Read the model definition and answer for the solid it produces. Units are mm, in the model's axes. A direction names the side the tool comes from. Give positions to 0.01 mm unless a question says otherwise; leave off trailing zeros. Write each loop counter-clockwise with the first axis right and the second up, starting at its lowest first coordinate (ties: lowest second). Pieces come first, ordered by that corner, then holes. Notation, with made-up numbers: M 51.25,-12 L 62.25,-12 A24 cw 62.25,26 Z; hole C 20.25,2 d3. An arc over 180 degrees is marked long. Use a Markdown table: item, result. Add a question column.
Item 1: Consider probe 1 along X at (y, z) = (-6.5, -1.25); probe 2 along X at (y, z) = (-8.5, 7); probe 3 along Y at (x, z) = (-1.5, 10.75) (3 decimals). Determine where each line is inside the solid, lowest interval first. Write a range as [from, to].
Item 2: A cutting plane is placed at B-B on y = 0. Determine the outline of the cut face in (x, z) (3 decimals).
Item 3: A cutting plane is placed at D-D on x = 9. Determine the outline of the cut face in (y, z).
Item 4: For faces 1 (the flat face through (0, -5, 0)), 2 (the flat face through (56.134, 9, -6)), 3 (the flat face through (66.294, 0, 0)), determine the directions among +Z, -Z, +X, -X, +Y, -Y from which every point of the face is accessible in a straight line to the end or side of a thin tool.
Item 5: A cutting plane is placed at C-C on x = -6.5. Determine the outline of the cut face in (y, z) (3 decimals).
Item 6: A cutting plane is placed at A-A on z = 0. Determine the outline of the cut face in (x, y) (3 decimals).
Item 7: Given P1, Ø6, axis at x = 8, z = 1.5, coming from the -Y side; P2, Ø5, axis at x = 40, y = -9, coming from the -Z side; P3, Ø12, axis at x = 10.5, y = 9.5, coming from the -Z side; P4, Ø3, axis at y = -7, z = 11.5, coming from the -X side, each flat-ended and moving along its own axis, determine where each tip first touches the part or whether it passes through.
Item 8: The mould has two halves that part along X. Classify faces 4 (the flat face through (-4.149, -0.044, -6.626)), 5 (the cylindrical face through (60.52, -12.4, -2.75)), 6 (the cylindrical face through (-3.626, 0.044, 0.954)): pulls with the +X half, pulls with the -X half, needs draft (parallel to the pull), parting line crosses it, or undercut.
from build123d import *

# Parameters (mm, degrees)
F0_W     = 5.842
F0_H     = 12.7
F0_R     = 3.175
F2_DEPTH = 3.175
F3_R     = 1.27


with BuildPart() as f1:
    # F0 (on Front) → F1 (revolve)
    with BuildSketch(Plane.XZ):
        with Locations((2.921, 6.35)):
            Rectangle(F0_W, F0_H)
        Polygon((5.842, 12.7), (5.842, 0), (66.294, 0), (66.294, 12.7), (56.134, 12.7), (56.134, 10.16), (10.16, 10.16), (10.16, 12.7), align=None)
    revolve(axis=Axis((33.147, 0, 0), (-1, 0, 0)))

    # F0 (on Front) → F2 (join, symmetric)
    with BuildSketch(Plane.XZ):
        with BuildLine():
            Line((-0.9398, 0), (0, 0))
            Line((0, 0), (0, 12.7))
            Line((0, 12.7), (5.842, 12.7))
            Line((5.842, 12.7), (5.842, 15.24))
            Line((5.842, 15.24), (-0.508, 15.24))
            Line((-0.508, 15.24), (-10.88063, 3.847543))
            ThreePointArc((-10.88063, 3.847543), (-4.591961, 5.329721), (-0.9398, 0))
        make_face()
        with BuildLine():
            ThreePointArc((-8.182663, -5.506983), (-3.195791, -4.549339), (-0.9398, 0))
            ThreePointArc((-0.9398, 0), (-4.591961, 5.329721), (-10.88063, 3.847543))
            ThreePointArc((-10.88063, 3.847543), (-12.145978, -1.583727), (-8.182663, -5.506983))
        make_face()
        with Locations((-6.6548, 0)):
            Circle(F0_R, mode=Mode.SUBTRACT)
        with BuildLine():
            Line((5.842, 0), (0, 0))
            Line((0, 0), (-0.9398, 0))
            ThreePointArc((-0.9398, 0), (-3.195791, -4.549339), (-8.182663, -5.506983))
            Line((-8.182663, -5.506983), (5.842, -9.398))
            Line((5.842, -9.398), (5.842, 0))
        make_face()
        with Locations((2.921, 6.35)):
            Rectangle(F0_W, F0_H)
    extrude(amount=F2_DEPTH, both=True)

    # F3
    f3_edges = [f1.edges().sort_by_distance(p)[0] for p in [
        (66.294, 0, -12.7),
    ]]
    fillet(f3_edges, radius=F3_R)


solid = f1.part
Filled in:
| question | item | result |
|---|---|---|
| 1 | probe 1 | [0, 66.29] |
| 1 | probe 2 | [0, 10.16], [56.13, 66.29] |
| 1 | probe 3 | [-3.175, 3.175] |
| 2 | outline | M -10.881,3.848 A5.715 ccw -8.183,-5.507 L 0,-7.777 L 0,-12.7 L 10.16,-12.7 L 10.16,-10.16 L 56.134,-10.16 L 56.134,-12.7 L 65.024,-12.7 A1.27 ccw 66.294,-11.43 L 66.294,11.43 A1.27 ccw 65.024,12.7 L 56.134,12.7 L 56.134,10.16 L 10.16,10.16 L 10.16,12.7 L 5.842,12.7 L 5.842,15.24 L -0.508,15.24 Z; hole C -6.655,0 d6.35 |
| 3 | outline | C 0,0 d25.4 |
| 4 | face 1 | -Z, -X |
| 4 | face 2 | none |
| 4 | face 3 | +Z, -Z, +X, +Y, -Y |
| 5 | outline | M -3.175,-5.974 L 3.175,-5.974 L 3.175,-3.171 L -3.175,-3.171 Z; M -3.175,3.171 L 3.175,3.171 L 3.175,8.659 L -3.175,8.659 Z |
| 6 | outline | M -12.37,-3.175 L -9.83,-3.175 L -9.83,3.175 L -12.37,3.175 Z; M -3.48,-3.175 L 0,-3.175 L 0,-12.7 L 10.16,-12.7 L 10.16,-10.16 L 56.134,-10.16 L 56.134,-12.7 L 65.024,-12.7 A1.27 ccw 66.294,-11.43 L 66.294,11.43 A1.27 ccw 65.024,12.7 L 56.134,12.7 L 56.134,10.16 L 10.16,10.16 L 10.16,12.7 L 0,12.7 L 0,3.175 L -3.48,3.175 Z |
| 7 | P1 | y = -12.7 |
| 7 | P2 | z = -7.81 |
| 7 | P3 | z = -12.21 |
| 7 | P4 | x = 0 |
| 8 | face 4 | pulls with the -X half |
| 8 | face 5 | needs draft |
| 8 | face 6 | undercut |
